Autodesk Inventor part; units mm, degrees
ref_plane "YZ Plane" through (0, 0, 0) normal (1, 0, 0) x (0, 1, 0)
ref_plane "XZ Plane" through (0, 0, 0) normal (0, 1, 0) x (-1, 0, 0)
ref_plane "XY Plane" through (0, 0, 0) normal (0, 0, 1) x (1, 0, 0)
sketch "Sketch1" plane through (0, 0, 0) normal (1, 0, 0) x (0, 1, 0)
  circle A0 centre (0, 0) radius 4.445
  circle A1 centre (0, 0) radius 8.255
  dimension "d0" = 8.89
  dimension "d1" = 3.81
extrude "Extrusion1" add sketch "Sketch1" along normal blind 19.812
sketch "Sketch2" plane through (0, 0, 0) normal (-1, 0, 0) x (0, 0, 1)
  circle A0 centre (0, 0) radius 8.255
  circle A1 centre (0, 0) radius 7.747
  circle A2 centre (0, 0) radius 8.255
  dimension "d42" = 0
extrude "Extrusion2" add sketch "Sketch2" along normal blind 2.54 contours A0 | A1
sketch "Sketch3" plane through (-2.54, 0, 0) normal (-1, 0, 0) x (0, 0, 1)
  line L0 (19.05, 48.5955) -> (-19.05, 48.5955)
  circle A0 centre (0, 0) radius 8.255
  line L1 (8.255, 0) -> (19.05, 48.5955)
  line L2 (-8.255, 0) -> (-19.05, 48.5955)
  arc A1 (8.255, 0) -> (-8.255, 0) centre (0, 0) ccw
  line L3 (-14.3008, 44.7855) -> (14.3008, 44.7855)
  line L4 (14.3008, 44.7855) -> (6.5962, 10.1022)
  arc A2 (6.5962, 10.1022) -> (-6.5962, 10.1022) centre (0, 0) ccw
  line L5 (-6.5962, 10.1022) -> (-14.3008, 44.7855)
  dimension "d6" = 38.1
  dimension "d7" = 19.05
  dimension "d8" = 3.81
extrude "Extrusion3" add sketch "Sketch3" against normal blind 6.35 contours L1 A0 L2 L0
sketch "Sketch6" plane through (-2.54, 44.7855, -14.3008) normal (0, -1, 0) x (1, 0, 0)
  line L0 (6.35, 32.4159) -> (26.9875, 32.4159)
  line L1 (13.4874, 32.4159) -> (13.4874, 26.0989)
  line L2 (26.9875, 32.4159) -> (26.9875, -3.9117)
  point P0 (2.54, 14.3008)
  dimension "d20" = 13.5001
sketch "Sketch10" plane through (0, 0, 0) normal (1, 0, 0) x (0, 0, -1)
  circle A0 centre (0, 0) radius 1.4542
  line L0 (-4.445, 1.4542) -> (4.445, 1.4542)
  line L1 (4.445, 1.4542) -> (4.445, -1.4542)
  line L2 (4.445, -1.4542) -> (-4.445, -1.4542)
  line L3 (-4.445, -1.4542) -> (-4.445, 1.4542)
  circle A1 centre (0, 0) radius 4.445
  dimension "d43" = 0
  dimension "d44" = 0
extrude "Extrusion7" cut sketch "Sketch10" against normal blind 22.225 contours A0 | A0 L0 A1 L2 | A0 L2 A1 L0 | A1 L3 L0 | L0 L1 A1 | A1 L1 L2 | L2 L3 A1
sketch "Sketch13" plane through (-2.54, 48.5955, 19.05) normal (0, 1, 0) x (1, 0, 0)
  line L0 (4.6355, 36.83) -> (1.7145, 36.83)
  line L1 (1.7145, 36.83) -> (1.7145, 33.909)
  line L2 (1.7145, 33.909) -> (4.6355, 33.909)
  line L3 (4.6355, 33.909) -> (4.6355, 36.83)
  line L4 (6.35, 38.1) -> (6.35, 0)
  line L5 (0, 38.1) -> (6.35, 38.1)
  line L6 (4.6228, 4.191) -> (1.7018, 4.191)
  line L7 (1.7018, 4.191) -> (1.7018, 1.27)
  line L8 (1.7018, 1.27) -> (4.6228, 1.27)
  line L9 (4.6228, 1.27) -> (4.6228, 4.191)
  line L10 (0, 0) -> (6.35, 0)
  line L11 (0, 0) -> (0, 38.1)
  line L12 (0, 0) -> (6.35, 0)
  line L13 (6.35, 38.1) -> (6.35, 0)
  line L14 (0, 38.1) -> (6.35, 38.1)
  point P0 (2.54, 19.05)
  dimension "d32" = 2.921
  dimension "d33" = 2.921
  dimension "d34" = 1.7145
  dimension "d35" = 1.27
  dimension "d36" = 2.921
  dimension "d37" = 2.921
  dimension "d38" = 1.7272
  dimension "d39" = 1.27
extrude "Extrusion9" add sketch "Sketch13" along normal blind 3.81 contours L3 L2 L1 L0 | L4 L10 L11 L5 | L9 L8 L7 L6
sketch "Sketch14" plane through (0, 0, 0) normal (-1, 0, 0) x (0, 0, 1)
  arc A0 (4.2004, -1.4542) -> (4.445, 0) centre (0, 0) ccw
  line L0 (4.2004, -1.4542) -> (4.445, -1.4542)
  line L1 (4.445, -1.4542) -> (4.445, 0)
  arc A1 (4.445, 0) -> (4.2004, 1.4542) centre (0, 0) ccw
  line L2 (4.445, 0) -> (4.445, 1.4542)
  line L3 (4.445, 1.4542) -> (4.2004, 1.4542)
  arc A2 (-4.445, 0) -> (-4.2004, -1.4542) centre (0, 0) ccw
  line L4 (-4.445, 0) -> (-4.445, -1.4542)
  line L5 (-4.445, -1.4542) -> (-4.2004, -1.4542)
  arc A3 (-4.2004, 1.4542) -> (-4.445, 0) centre (0, 0) ccw
  line L6 (-4.2004, 1.4542) -> (-4.445, 1.4542)
  line L7 (-4.445, 1.4542) -> (-4.445, 0)
extrude "Extrusion10" add sketch "Sketch14" along normal blind 2.54
sketch "Sketch15" plane through (-2.54, 0, 0) normal (-1, 0, 0) x (0, 0, 1)
  circle A0 centre (0, 0) radius 41.275
  circle A1 centre (0, 0) radius 44.45
  dimension "d47" = 82.55
  dimension "d48" = 88.9
extrude "Extrusion11" add sketch "Sketch15" against normal blind 2.54
sketch "Sketch16" plane through (0, 0, 0) normal (1, 0, 0) x (0, 0, -1)
  circle A0 centre (0, 0) radius 44.45
  circle A1 centre (0, 0) radius 41.275
  dimension "d51" = 82.55
extrude "Extrusion12" add sketch "Sketch16" along normal blind 38.1
sketch "Sketch19" plane through (-2.54, 0, 0) normal (-1, 0, 0) x (0, 0, 1)
  line L0 (4.2004, 1.4542) -> (-4.2004, 1.4542)
  arc A0 (-16.6452, 37.7699) -> (16.6452, 37.7699) centre (0, 0) ccw
  line L1 (-4.2004, 1.4542) -> (-41.2494, 1.4542)
  line L2 (4.2004, 1.4542) -> (41.2494, 1.4542)
  circle A1 centre (0, 0) radius 8.382
  line L3 (-4.2004, -1.4542) -> (4.2004, -1.4542)
  line L4 (4.2004, 1.4542) -> (-4.2004, 1.4542)
  line L5 (-41.2494, -1.4542) -> (41.2494, -1.4542)
extrude "Extrusion14" add sketch "Sketch19" against normal blind 6.35 contours L2 A1 L5 L3 L1 L0 | L2 A0 L5 A1 | A1 L5 A0 L1
sketch "Sketch20" plane through (3.81, 0, 0) normal (1, 0, 0) x (0, 0, -1)
  arc A0 (4.2004, -1.4542) -> (4.2004, 1.4542) centre (0, 0) ccw
  line L0 (4.2004, 1.4542) -> (-4.2004, 1.4542)
  arc A1 (-4.2004, 1.4542) -> (-4.2004, -1.4542) centre (0, 0) ccw
  line L1 (-4.2004, -1.4542) -> (4.2004, -1.4542)
extrude "Extrusion15" cut sketch "Sketch20" against normal blind 6.35
sketch "Sketch21" plane through (-2.54, 0, 0) normal (-1, 0, 0) x (0, 0, 1)
  arc A0 (-8.1259, -1.4542) -> (8.1259, -1.4542) centre (0, 0) ccw
  line L0 (1.8212, -8.0516) -> (1.8212, -41.2348)
  arc A1 (-41.2494, -1.4542) -> (41.2494, -1.4542) centre (0, 0) ccw
  line L1 (-1.8492, -41.2336) -> (-1.8492, -8.1755)
  arc A2 (-1.8492, -41.2336) -> (1.8212, -41.2348) centre (0, 0) ccw
  line L2 (-1.8492, -8.1755) -> (-1.8492, -8.0452)
extrude "Extrusion16" add sketch "Sketch21" against normal blind 6.35
sketch "Sketch23" plane through (3.81, 0, 0) normal (1, 0, 0) x (0, 0, -1)
  line L0 (19.05, 52.4055) -> (-19.05, 52.4055)
  line L1 (-19.05, 48.5955) -> (-19.05, 52.4055)
  line L2 (19.05, 52.4055) -> (-19.05, 52.4055)
  line L3 (-19.05, 52.4055) -> (-19.05, 48.5955)
  line L4 (-19.05, 48.5955) -> (19.05, 48.5955)
  line L5 (19.05, 48.5955) -> (19.05, 52.4055)
  point P0 (0, 0)
extrude "Extrusion17" add sketch "Sketch23" along normal blind 19.05
properties part number "BasicThrustMotorHousing"
Work out the finished part from the listing and answer in its coordinate system (mm). A direction names the side the tool comes from. Give positions to 0.01 mm unless a question says otherwise; leave off trailing zeros. Loops run counter-clockwise (first coordinate to the right, second up) from the corner with the lowest first, then second, coordinate; pieces in that order, holes last. Notation, with made-up numbers: (40.5, 24.5) - (47.5, 24.5) arc R10 cw to (47.5, 37.5) - close; hole circle Ø10 at (34.25, 61.5). An arc over 180 degrees is marked (long way). One line per question, with ' | ' between items.
(1) The part is cut by section A-A (x = 5.5). Count the separate pieces of the cut face and the enclosed holes in it, then the cut area to 3 significant figures.
Recorded:
separate pieces: 3 | enclosed holes: 2 | area: 1,150 mm²
(2) The mould has two halves that part along Y. Classify faces 4 (the face through (-2.54, 4, 0)), 5 (the face through (10, 52.406, 0)), 6 (the face through (10.963, -6.551, 5.023)): +Y half, -Y half, draft (parallel to the pull), parting line (faces both ways), or undercut.
Recorded:
face 4: draft | face 5: +Y half | face 6: undercut
(3) Each of these flat-tipped pins is pushed along its axis until it touches: pin 1 Ø2 at (x, z) = (29, 17.5) entering from -Y; pin 2 Ø7 at (x, y) = (0, -25) entering from -Z; pin 3 Ø1.5 at (x, z) = (5, -22.5) entering from -Y; pin 4 Ø6 at (y, z) = (29, 22) entering from +X. Where does it stop, or does it pass through?
Recorded:
pin 1: stops at y = -41.27 | pin 2: stops at z = -38.9 | pin 3: stops at y = -38.77 | pin 4: passes through
(4) A tool of negligible diameter and unlimited length cuts with its end or side. For faces 1 (the face through (13, 48.596, 0)), 2 (the face through (-1, -1.454, 0)), 3 (the face through (22.86, 51, 0)), from which of +Z, -Z, +X, -X, +Y, -Y can it reach the whole face along a straight path? Write none if from no direction.
Recorded:
face 1: +Z, -Z, +X | face 2: +X, -X | face 3: +Z, -Z, +X, +Y
(5) The part is cut by section C-C (y = -23.5). Write down the section's boundary in (x, z).
Recorded:
outline: (-2.54, -37.73) - (38.1, -37.73) - (38.1, -33.93) - (-2.54, -33.93) - close; (-2.54, -1.85) - (3.81, -1.85) - (3.81, 1.82) - (-2.54, 1.82) - close; (-2.54, 33.93) - (38.1, 33.93) - (38.1, 37.73) - (-2.54, 37.73) - close
(6) Straight lines are drawn through the part: probe 1 along Z at (x, y) = (29, 0) (3 decimals); probe 2 along Z at (x, y) = (12, -3). For each, find the intervals that lie inside material, in ascending order.
Recorded:
probe 1: z = -44.45 to -41.275, 41.275 to 44.45 | probe 2: z = -44.35 to -41.17, -7.69 to -3.28, 3.28 to 7.69, 41.17 to 44.35
